```python
from build123d import *

# Parameters (mm, degrees)
SKETCH1_R           = 92.075
BOSS_EXTRUDE1_DEPTH = 50.8
SKETCH6_W           = 27.94
SKETCH6_H           = 27.94
CUT_EXTRUDE4_DEPTH  = 50.8
CUT_EXTRUDE5_DEPTH  = 50.8
SKETCH10_W          = 7.5
SKETCH10_H          = 73
CUT_EXTRUDE7_DEPTH  = 15.24


with BuildPart() as part:
    # Sketch1 → Boss-Extrude1 (new body)
    with BuildSketch(Plane(origin=(0, 0, 0), x_dir=(1, 0, 0), z_dir=(0, 1, 0))):
        with Locations(Location((0, 0, 0), (0, 0, 270))):
            Circle(SKETCH1_R)
    extrude(amount=BOSS_EXTRUDE1_DEPTH)

    # Sketch6 → Cut-Extrude4 (cut)
    with BuildSketch(Plane.XZ):
        with Locations((30.48, 49.53)):
            Rectangle(SKETCH6_W, SKETCH6_H)
        with Locations((-30.48, 49.53)):
            Rectangle(SKETCH6_W, SKETCH6_H)
    extrude(amount=-CUT_EXTRUDE4_DEPTH, mode=Mode.SUBTRACT)

    # Sketch8 → Cut-Extrude5 (cut)
    with BuildSketch(Plane(origin=(0, 50.8, 0), x_dir=(1, 0, 0), z_dir=(0, 1, 0))):
        Polygon((48.673227998, 66.920620093), (48.673227998, 31.675), (53.066023648, 31.675), (53.066023648, 30.175), (51.568299971, 30.175), (51.568299971, -2.285), (49.028299971, -4.825), (32.568299971, -4.825), (32.568299971, -24.825), (28.568299971, -24.825), (28.568299971, -4.825), (12.108299971, -4.825), (9.568299971, -2.285), (9.568299971, 30.175), (8.06602381, 30.175), (8.06602381, 31.675), (10.838299971, 31.675), (11.658892904, 31.675), (11.658892904, 66.920620093), (11.658892904, 71.12), (48.673227998, 71.12), align=None)
        Polygon((-8.831700029, -2.285), (-11.371700029, -4.825), (-27.831700029, -4.825), (-27.831700029, -24.825), (-31.831700029, -24.825), (-31.831700029, -4.825), (-48.291700029, -4.825), (-50.831700029, -2.285), (-50.831700029, 30.175), (-52.33397619, 30.175), (-52.33397619, 31.675), (-48.741107096, 31.675), (-48.741107096, 66.920620093), (-48.741107096, 71.12), (-11.726772002, 71.12), (-11.726772002, 66.920620093), (-11.726772002, 31.675), (-7.333976352, 31.675), (-7.333976352, 30.175), (-8.831700029, 30.175), align=None)
    extrude(amount=-CUT_EXTRUDE5_DEPTH, mode=Mode.SUBTRACT)

    # Sketch10 → Cut-Extrude7 (cut)
    with BuildSketch(Plane(origin=(0, 50.8, 0), x_dir=(1, 0, 0), z_dir=(0, 1, 0))):
        with Locations((70.806, 0)):
            Rectangle(SKETCH10_W, SKETCH10_H)
    extrude(amount=-CUT_EXTRUDE7_DEPTH, mode=Mode.SUBTRACT)


solid = part.part
```
Geometry: final body of the model. Coordinates: model frame, mm. A direction names the side the tool comes from. Coordinates: 2 decimals unless noted, no trailing zeros. Loops run counter-clockwise (first coordinate to the right, second up) from the corner with the lowest first, then second, coordinate; pieces in that order, holes last. Notation, with made-up numbers: M -14.75,-8.5 L 38.25,-8.5 A20 ccw 38.25,19.5 Z; hole C -27,54.5 d11. An arc over 180 degrees is marked long. Put each result on its own line as item: value.
(1) Access query for faces 4 (the face through (28.568, 26, 15)), 5 (the face through (71, 35.56, -1)), 6 (the face through (1, 50.8, -1)). Directions: +Z, -Z, +X, -X, +Y, -Y. A direction counts if a zero-diameter tool reaches every point of the face in a straight line with its end or side. Return the directions, or none.
Answer sheet:
face 4: +Y, -Y
face 5: +Y
face 6: +Z, -Z, +X, -X, +Y
(2) Cut plane D-D on z = 29. Return the cut outline in (x, y), then the cut area to 3 significant figures.
Answer sheet:
outline: M -87.39,0 L 87.39,0 L 87.39,50.8 L 74.56,50.8 L 74.56,35.56 L 67.06,35.56 L 67.06,50.8 L -87.39,50.8 Z
area: 8,760 mm^2
(3) Cut plane B-B on x = 70. Return the cut outline in (y, z), then the cut area to 3 significant figures.
Answer sheet:
outline: M 0,-59.81 L 50.8,-59.81 L 50.8,-36.5 L 35.56,-36.5 L 35.56,36.5 L 50.8,36.5 L 50.8,59.81 L 0,59.81 Z
area: 4,960 mm^2
(4) Cut plane A-A on z = 0. Return the cut outline in (x, y) (3 decimals), then the cut area to 3 significant figures.
Answer sheet:
outline: M -92.075,0 L -50.832,0 L -50.832,50.8 L -92.075,50.8 Z; M -8.832,0 L 9.568,0 L 9.568,50.8 L -8.832,50.8 Z; M 51.568,0 L 92.075,0 L 92.075,50.8 L 74.556,50.8 L 74.556,35.56 L 67.056,35.56 L 67.056,50.8 L 51.568,50.8 Z
area: 4,970 mm^2
(5) Cut plane C-C on y = 8. State how many separate pieces and enclosed holes the cut face has, then the cut area to 3 significant figures.
Answer sheet:
separate pieces: 1
enclosed holes: 4
area: 18,900 mm^2
(6) Material intervals for probe 1 along X at (y, z) = (25.5, -69); probe 2 along Z at (x, y) = (43, 12) (3 decimals); probe 3 along X at (y, z) = (3, 41.5), sorted ascending.
Answer sheet:
probe 1: x = -60.97 to -48.74, -11.73 to 11.66, 48.67 to 60.97
probe 2: z = -81.417 to -71.12, 4.825 to 35.56, 63.5 to 81.417
probe 3: x = -82.19 to -44.45, -16.51 to 16.51, 44.45 to 82.19
(7) First-contact query: pin 1 (4 mm diameter, centred on x = 34, z = 38.5, fed in from +Y); pin 2 (8.5 mm diameter, centred on y = 20, z = 43.5, fed in from -X); pin 3 (2 mm diameter, centred on y = 20, z = -63, fed in from -X); pin 4 (1.1 mm diameter, centred on x = -51, y = 33, fed in from +Z). Flat tips, straight axial feed; report the tip coordinate or a pass-through.
Answer sheet:
pin 1: passes through
pin 2: stops at x = -83.29
pin 3: stops at x = -68.07
pin 4: stops at z = 77.02
(8) Draft query along X for faces 1 (the face through (71, 43, 36.5)), 2 (the face through (-89.885, 25.044, -19.96)), 3 (the face through (1, 0, -1)). Return one class per face: pulls with the +X half, pulls with the -X half, needs draft (parallel to the pull), parting line crosses it, or undercut.
Answer sheet:
face 1: undercut
face 2: parting line crosses it
face 3: needs draft
